Verification items for the finished model (mm, model axes). Face numbers are marked on the shaded views. A direction names the side the tool comes from. Give positions to 0.01 mm unless a question says otherwise; leave off trailing zeros. Write each loop counter-clockwise with the first axis right and the second up, starting at its lowest first coordinate (ties: lowest second). Pieces come first, ordered by that corner, then holes. Notation, with made-up numbers: (-31, 42) - (-10, 42) arc R21 ccw to (-10, 70) - close; hole circle Ø10 at (13, -31). An arc over 180 degrees is marked (long way). Answer as a JSON object with one key per item and string values. Group by question number.
Item 1: Go/stop test with flat-tipped pins: pin 1 (3 mm diameter, centred on x = 346.5, z = -76.5, fed in from +Y); pin 2 (1.5 mm diameter, centred on x = 335.5, y = 51.5, fed in from +Z); pin 3 (3 mm diameter, centred on x = 453, z = -322.5, fed in from +Y). Record where each tip stops, or that it passes through.
Item 2: Sectioned sample at A-A, the plane x = 118. Record the boundary of the cut face in (y, z), and give its area (4 significant figures).
Item 3: Scan lines: line 1 along Y through (x, z) = (125.5, -442); line 2 along Z through (x, y) = (526, 52.5); line 3 along Y through (x, z) = (121, -95.5). Record each from-to range of solid material in increasing order. Write a range as [from, to].
Item 4: Tool access check on the marked faces 1, 2 and 3. Record the directions out of +Z, -Z, +X, -X, +Y, -Y that give a thin tool (end or side, any length) a straight path to the whole face; none if there is none.
Item 5: Sectioned sample at B-B, the plane y = 62. Record the boundary of the cut face in (x, z).
Item 6: Sectioned sample at C-C, the plane z = -234. Record the boundary of the cut face in (x, y).
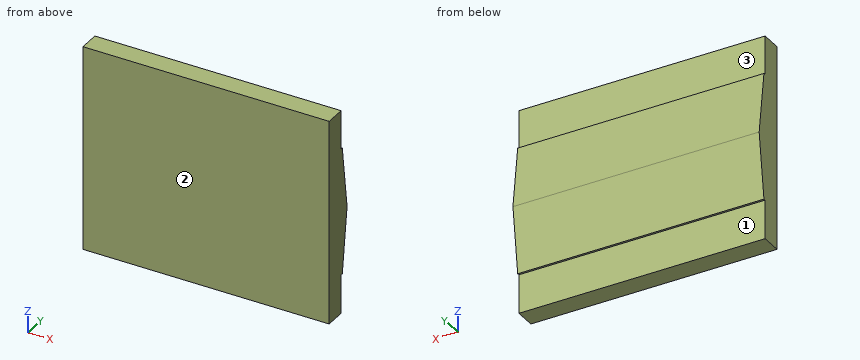
```python
from build123d import *

# Parameters (mm, degrees)
SKETCH_1_W          = 600
SKETCH_1_H          = 500
EXTRUDE_1_DEPTH     = 75
CUT_EXTRUDE_1_DEPTH = 785.617741324
CUT_EXTRUDE_2_DEPTH = 785.617741324


with BuildPart() as part:
    # 草图1 → 凸台-拉伸1 (new body)
    with BuildSketch(Plane(origin=(0, 0, 0), x_dir=(1, 0, 0), z_dir=(0, 1, 0))):
        with Locations((300, 250)):
            Rectangle(SKETCH_1_W, SKETCH_1_H)
    extrude(amount=EXTRUDE_1_DEPTH)

    # 草图3 → 切除-拉伸1 (cut, through all)
    with BuildSketch(Plane(origin=(600, 0, 0), x_dir=(0, 0, -1), z_dir=(1, 0, 0))):
        Polygon((405, 55), (405, 50), (500, 50), (500, 75), (250, 75), align=None)
    extrude(amount=-CUT_EXTRUDE_1_DEPTH, mode=Mode.SUBTRACT)

    # 草图4 → 切除-拉伸2 (cut, through all)
    with BuildSketch(Plane(origin=(600, 0, 0), x_dir=(0, 0, -1), z_dir=(1, 0, 0))):
        Polygon((0, 75), (0, 50), (95, 50), (95, 55), (250, 75), align=None)
    extrude(amount=-CUT_EXTRUDE_2_DEPTH, mode=Mode.SUBTRACT)


solid = part.part
```
Geometry check:
{
 "1": {"pin 1": "y = 50", "pin 2": "z = -95", "pin 3": "y = 65.84"},
 "2": {"outline": "(0, -500) - (50, -500) - (50, -405) - (55, -405) - (75, -250) - (55, -95) - (50, -95) - (50, 0) - (0, 0) - close", "area": "29,650 mm^2"},
 "3": {"line 1": "[0, 50]", "line 2": "[-405, -95]", "line 3": "[0, 55.06]"},
 "4": {"face 1": "-Z, +X, -X, +Y", "face 2": "+Z, -Z, +X, -X, -Y", "face 3": "+Z, +X, -X, +Y"},
 "5": {"outline": "(0, -350.75) - (600, -350.75) - (600, -149.25) - (0, -149.25) - close"},
 "6": {"outline": "(0, 0) - (600, 0) - (600, 72.94) - (0, 72.94) - close"}
}
